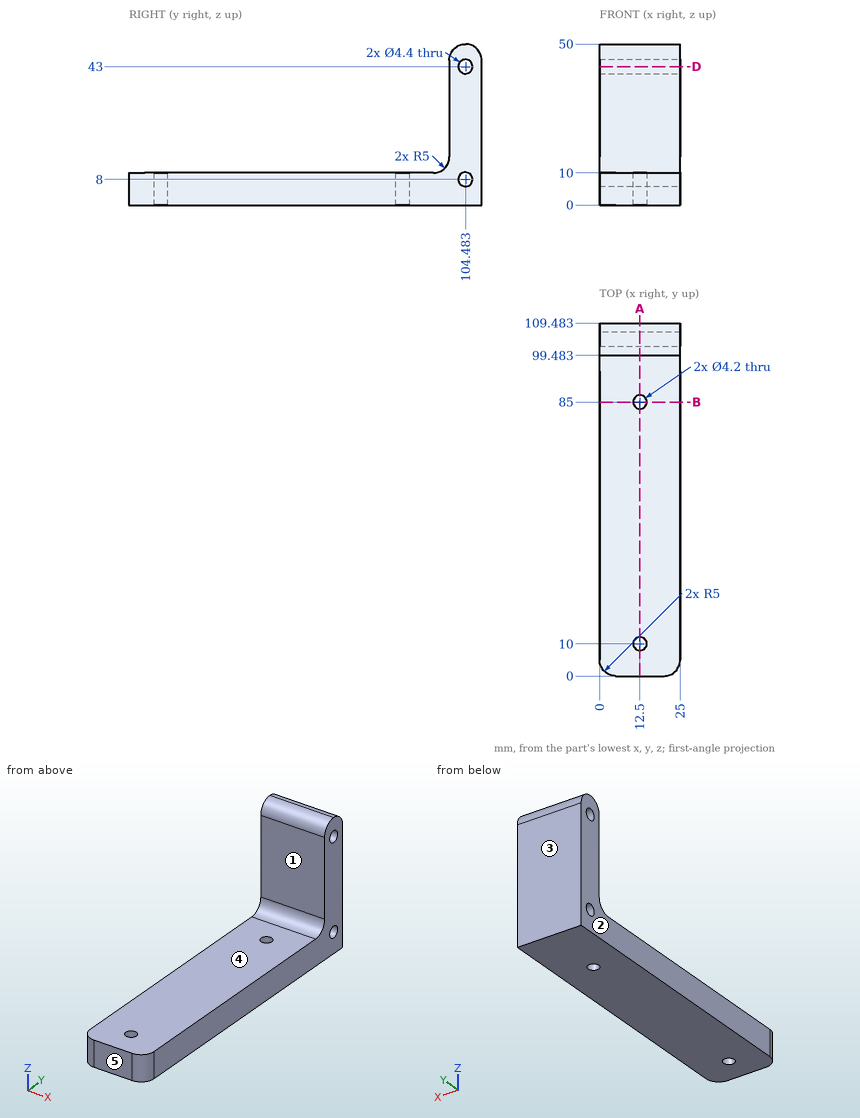
Study the drawing (mm; zero at the part's minimum x, y, z) and answer. A direction names the side the tool comes from. Give positions to 0.01 mm unless a question says otherwise; leave off trailing zeros. Loops run counter-clockwise (first coordinate to the right, second up) from the corner with the lowest first, then second, coordinate; pieces in that order, holes last. Notation, with made-up numbers: (21.5, 29.5) - (29.5, 29.5) arc R27 ccw to (29.5, 63.5) - close; hole circle Ø11 at (30, 86). An arc over 180 degrees is marked (long way). Return JSON: item names as keys, results as strings. Group by question number.
1. Which of the six approach directions +Z, -Z, +X, -X, +Y, -Y give full straight-line access (tool end or side, diameter ignored) to the marked faces 1 and 2?
2. Find section A-A (x = 12.5). State how many separate pieces and enclosed holes the cut face has, then the cut area to 4 significant figures.
3. Given pin 1 Ø1.5 at (x, z) = (14, 45) entering from -Y; pin 2 Ø3 at (x, y) = (2.5, 73) entering from +Z, each flat-ended and moving along its own axis, determine where each tip first touches the part or whether it passes through.
4. Find section D-D (z = 43). Write down the section's boundary in (x, y).
5. Determine the mould class of the marked faces 3, 4 and 5 for opening direction Y: pulls with the +Y half, pulls with the -Y half, needs draft (parallel to the pull), parting line crosses it, or undercut.
6. Straight lines are drawn through the part: line 1 (Y direction, x = 12.5, z = 5); line 2 (Y direction, x = 12.5, z = 6.5); line 3 (Z direction, x = 17.5, y = 82.5). For each, find the intervals that lie inside material, in ascending order. Write a range as [from, to].
7. Find section B-B (y = 85). Write down the section's boundary in (x, z), then the cut area to 3 significant figures.
Verdict:
{
 "1": {"face 1": "+Z, +X, -X, -Y", "face 2": "+Z, -Z, -X, +Y, -Y"},
 "2": {"separate pieces": "3", "enclosed holes": "2", "area": "1,375 mm^2"},
 "3": {"pin 1": "stops at y = 99.48", "pin 2": "stops at z = 10"},
 "4": {"outline": "(0, 99.48) - (25, 99.48) - (25, 102.28) - (0, 102.28) - close; (0, 106.68) - (25, 106.68) - (25, 109.48) - (0, 109.48) - close"},
 "5": {"face 3": "pulls with the +Y half", "face 4": "needs draft", "face 5": "pulls with the -Y half"},
 "6": {"line 1": "y = [0, 7.9], [12.1, 82.9], [87.1, 109.48]", "line 2": "y = [0, 7.9], [12.1, 82.9], [87.1, 102.87], [106.09, 109.48]", "line 3": "z = [0, 10]"},
 "7": {"outline": "(0, 0) - (10.4, 0) - (10.4, 10) - (0, 10) - close; (14.6, 0) - (25, 0) - (25, 10) - (14.6, 10) - close", "area": "208 mm^2"}
}
